from build123d import *

# Parameters (mm, degrees)
SKETCH1_W           = 104.648
SKETCH1_H           = 130.048
BOSS_EXTRUDE1_DEPTH = 36.068
SKETCH2_W           = 15.494
SKETCH2_H           = 124.968
CUT_EXTRUDE1_DEPTH  = 129.375329032
SKETCH3_W           = 98.298
SKETCH3_H           = 93.853
CUT_EXTRUDE2_DEPTH  = 18.796
SKETCH4_W           = 86.36
SKETCH4_H           = 53.34
CUT_EXTRUDE3_DEPTH  = 18.796
CUT_EXTRUDE4_DEPTH  = 18.796


with BuildPart() as part:
    # Sketch1 → Boss-Extrude1 (new body)
    with BuildSketch(Plane.XY):
        Rectangle(SKETCH1_W, SKETCH1_H)
    extrude(amount=BOSS_EXTRUDE1_DEPTH)

    # Sketch2 → Cut-Extrude1 (cut, through all)
    with BuildSketch(Plane(origin=(52.324, 0, 0), x_dir=(0, 0, -1), z_dir=(1, 0, 0))):
        with Locations((-7.747, 2.54)):
            Rectangle(SKETCH2_W, SKETCH2_H)
    extrude(amount=-CUT_EXTRUDE1_DEPTH, mode=Mode.SUBTRACT)

    # Sketch3 → Cut-Extrude2 (cut)
    with BuildSketch(Plane(origin=(0, 0, 15.494), x_dir=(-1, 0, 0), z_dir=(0, 0, -1))):
        with Locations((0, 14.9225)):
            Rectangle(SKETCH3_W, SKETCH3_H)
    extrude(amount=-CUT_EXTRUDE2_DEPTH, mode=Mode.SUBTRACT)

    # Sketch4 → Cut-Extrude3 (cut)
    with BuildSketch(Plane.XY.offset(36.068)):
        with Locations((-0.637536215, 24.384)):
            Rectangle(SKETCH4_W, SKETCH4_H)
    extrude(amount=-CUT_EXTRUDE3_DEPTH, mode=Mode.SUBTRACT)

    # Sketch5 → Cut-Extrude4 (cut)
    with BuildSketch(Plane.XY.offset(36.068)):
        with BuildLine():
            ThreePointArc((43.47484815, -18.415), (36.997914828, -9.415751935), (26.407785194, -12.7))
            Line((26.407785194, -12.7), (40.558113562, -12.7))
            Line((40.558113562, -12.7), (40.558113562, -24.13))
            Line((40.558113562, -24.13), (26.407785194, -24.13))
            ThreePointArc((26.407785194, -24.13), (36.997914828, -27.414248065), (43.47484815, -18.415))
        make_face()
        with BuildLine():
            Line((40.558113562, -12.7), (26.407785194, -12.7))
            ThreePointArc((26.407785194, -12.7), (24.494085978, -18.415), (26.407785194, -24.13))
            Line((26.407785194, -24.13), (40.558113562, -24.13))
            Line((40.558113562, -24.13), (40.558113562, -12.7))
        make_face()
        with BuildLine():
            Line((26.407785194, -12.7), (-41.229886438, -12.7))
            Line((-41.229886438, -12.7), (-41.229886438, -24.13))
            Line((-41.229886438, -24.13), (26.407785194, -24.13))
            ThreePointArc((26.407785194, -24.13), (24.494085978, -18.415), (26.407785194, -12.7))
        make_face()
    extrude(amount=-CUT_EXTRUDE4_DEPTH, mode=Mode.SUBTRACT)


solid = part.part
Geometry check sheet. Reference: the model listing, model coordinates, mm. A direction names the side the tool comes from. Coordinates: 2 decimals unless noted, no trailing zeros. Write each loop counter-clockwise with the first axis right and the second up, starting at its lowest first coordinate (ties: lowest second). Pieces come first, ordered by that corner, then holes. Notation, with made-up numbers: (-36, 12) -> (-19, 12) arc R17 ccw to (-19, 38) -> close; hole circle Ø11 at (-7.75, -16.75). An arc over 180 degrees is marked (long way). One line per question, with ' | ' between items.
1. Draft check along X on faces 4 (the flat face through (52.324, -1, 26)), 5 (the flat face through (1, 61.849, 25)), 6 (the flat face through (-1, 65.024, 26)), 7 (the flat face through (49.149, 14, 25)). Enter one of: +X half, -X half, draft (parallel to the pull), parting line (faces both ways), or undercut.
Answers:
face 4: +X half | face 5: undercut | face 6: draft | face 7: undercut
2. Thickness scan on probe 1 along X at (y, z) = (-27.5, 31); probe 2 along Y at (x, z) = (-42.5, 23); probe 3 along Z at (x, y) = (5, -50). Record the ranges inside material, lowest first. Write a range as from..to.
Answers:
probe 1: x = -52.32..-49.15, 49.15..52.32 | probe 2: y = -65.02..-32, 61.85..65.02 | probe 3: z = 15.49..36.07
3. Cross-section at B-B on x = 9. Record the cut outline in (y, z).
Answers:
outline: (-65.02, 0) -> (-59.94, 0) -> (-59.94, 15.49) -> (-32, 15.49) -> (-32, 34.29) -> (-24.13, 34.29) -> (-24.13, 36.07) -> (-65.02, 36.07) -> close; (-12.7, 34.29) -> (-2.29, 34.29) -> (-2.29, 36.07) -> (-12.7, 36.07) -> close; (51.05, 34.29) -> (61.85, 34.29) -> (61.85, 15.49) -> (65.02, 15.49) -> (65.02, 36.07) -> (51.05, 36.07) -> close
4. Cross-section at A-A on y = 26. Record the cut outline in (x, z).
Answers:
outline: (-52.32, 15.49) -> (-49.15, 15.49) -> (-49.15, 34.29) -> (-43.82, 34.29) -> (-43.82, 36.07) -> (-52.32, 36.07) -> close; (42.54, 34.29) -> (49.15, 34.29) -> (49.15, 15.49) -> (52.32, 15.49) -> (52.32, 36.07) -> (42.54, 36.07) -> close
5. Cross-section at C-C on z = 28. Record the cut outline in (x, y).
Answers:
outline: (-52.32, -65.02) -> (52.32, -65.02) -> (52.32, 65.02) -> (-52.32, 65.02) -> close; hole (-49.15, -32) -> (49.15, -32) -> (49.15, 61.85) -> (-49.15, 61.85) -> close
6. Set-up check for faces 1 (the flat face through (12, -5, 34.29)), 2 (the flat face through (1, -59.944, 8)), 3 (the flat face through (-1, -28, 36.068)): record each of +Z, -Z, +X, -X, +Y, -Y from which the full face is reachable in a straight line by a thin tool's end or side.
Answers:
face 1: -Z | face 2: -Z, +X, -X, +Y | face 3: +Z, +X, -X, +Y, -Y
7. Depth check by flat-ended pin: pin 1 Ø10 at (x, z) = (29.5, 6.5) entering from +Y; pin 2 Ø5 at (x, y) = (-5.5, -27) entering from -Z. Enter the tip coordinate at first touch or a pass-through.
Answers:
pin 1: stops at y = -59.94 | pin 2: stops at z = 34.29
8. Cross-section at D-D on x = 39. Record the cut outline in (y, z).
Answers:
outline: (-65.02, 0) -> (-59.94, 0) -> (-59.94, 15.49) -> (-32, 15.49) -> (-32, 34.29) -> (-26.47, 34.29) -> (-26.47, 36.07) -> (-65.02, 36.07) -> close; (-10.36, 34.29) -> (-2.29, 34.29) -> (-2.29, 36.07) -> (-10.36, 36.07) -> close; (51.05, 34.29) -> (61.85, 34.29) -> (61.85, 15.49) -> (65.02, 15.49) -> (65.02, 36.07) -> (51.05, 36.07) -> close
